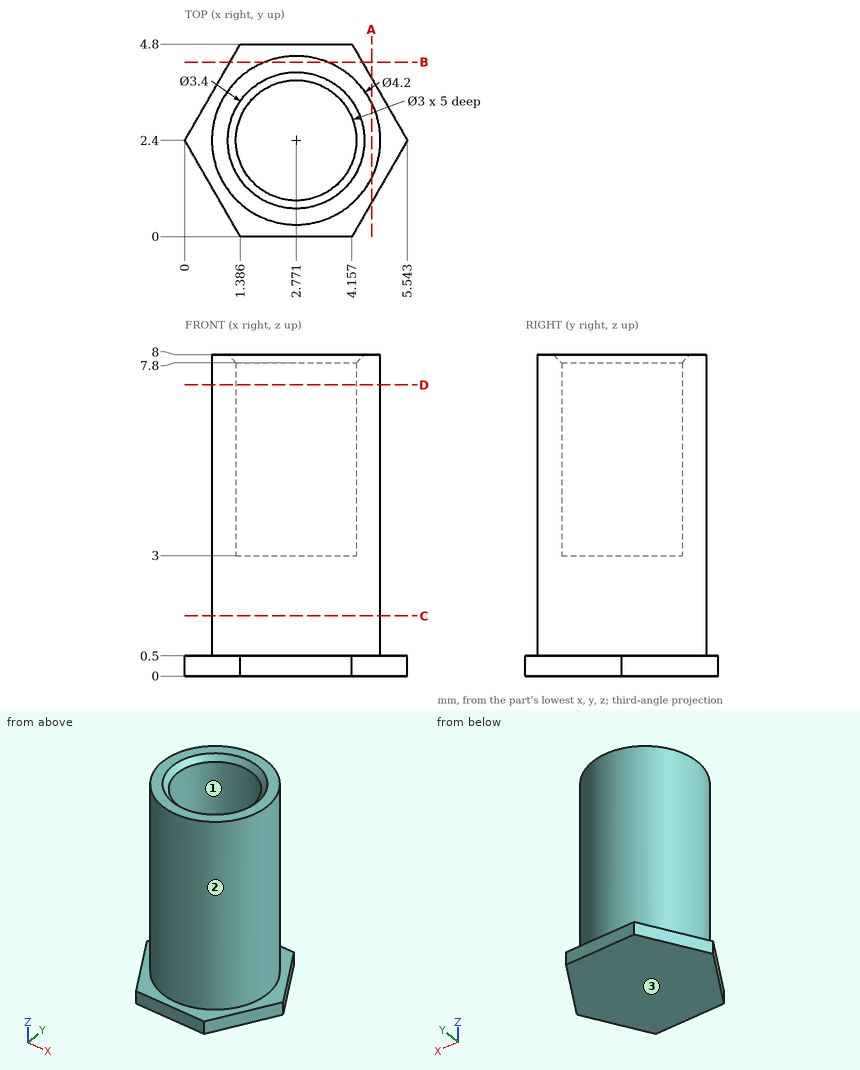
For this review, use the dimensioned drawing (mm, ordinates from the lowest corner) and the shaded views. Round coordinates to 2 decimals unless told otherwise and drop trailing zeros. Write each loop counter-clockwise with the first axis right and the second up, starting at its lowest first coordinate (ties: lowest second). Pieces come first, ordered by that corner, then holes. Notation, with made-up numbers: M 28.5,-15.5 L 34.5,-15.5 A25 cw 34.5,12.5 Z; hole C -10.5,-19 d4. An arc over 180 degrees is marked long. Answer as CSV lines item,"result". Start each with the question number.
Q1. Consider section B-B, the plane y = 4.35. Give the boundary of the cut face in (x, z).
Q2. Clearance check with flat-ended pins moving along their axes: P1, Ø2, axis at y = 1, z = 2.5, coming from the +X side; P2, Ø1.5, axis at x = 0.5, z = 3.5, coming from the -Y side; P3, Ø1.4, axis at x = 3, y = 1.5, coming from the +Z side; P4, Ø1.5, axis at x = 2, y = 3, coming from the +Z side. State where each tip first meets the part, or that it passes through.
Q3. Consider section A-A, the plane x = 4.65. Give the boundary of the cut face in (y, z), then the cut area to 3 significant figures.
Q4. Consider section D-D, the plane z = 7.25. Give the boundary of the cut face in (x, y).
Q5. The part is to be moulded in two halves that separate along X. For the marked faces 1, 2 and 3, say which applies: +X half, -X half, draft (parallel to the pull), parting line (faces both ways), or undercut.
Q6. Wall thickness on line 1 along Z through (x, y) = (4.95, 2.7); line 2 along Z through (x, y) = (2.25, 1.55); line 3 along Y through (x, z) = (2.3, 4) (1 decimal): over which ranges is each line inside the solid? List them lowest first.
Q7. Consider section C-C, the plane z = 1.5. Give the boundary of the cut face in (x, y).
Result set:
1,outline,"M 1.13,0 L 4.42,0 L 4.42,0.5 L 3.55,0.5 L 3.55,8 L 1.99,8 L 1.99,0.5 L 1.13,0.5 Z"
2,P1,"stops at x = 4.83"
2,P2,"stops at y = 0.95"
2,P3,"stops at z = 7.93"
2,P4,"stops at z = 8"
3,outline,"M 0.85,0 L 3.95,0 L 3.95,0.5 L 3.34,0.5 L 3.34,8 L 1.46,8 L 1.46,0.5 L 0.85,0.5 Z"
3,area,"15.6 mm²"
4,outline,"C 2.77,2.4 d4.2; hole C 2.77,2.4 d3"
5,face 1,"undercut"
5,face 2,"parting line"
5,face 3,"draft"
6,line 1,"z = 0 to 0.5"
6,line 2,"z = 0 to 3"
6,line 3,"y = 0.4 to 1, 3.8 to 4.4"
7,outline,"C 2.77,2.4 d4.2"
